```python
from build123d import *

# Parameters (mm, degrees)
SKETCH1_R           = 7.5
BOSS_EXTRUDE1_DEPTH = 300
CUT_EXTRUDE1_DEPTH  = 5


with BuildPart() as part:
    # Sketch1 → Boss-Extrude1 (new body)
    with BuildSketch(Plane.XY):
        with Locations((-21.928145629, 1.412024527)):
            Circle(SKETCH1_R)
    extrude(amount=BOSS_EXTRUDE1_DEPTH)

    # Sketch2 → Cut-Extrude1 (cut)
    with BuildSketch(Plane.XY.offset(300)):
        with BuildLine():
            Line((-23.928145629, 3.412024527), (-23.928145629, -0.587975473))
            ThreePointArc((-23.928145629, -0.587975473), (-21.928145629, -1.587975473), (-19.928145629, -0.587975473))
            Line((-19.928145629, -0.587975473), (-19.928145629, 3.412024527))
            ThreePointArc((-19.928145629, 3.412024527), (-21.928145629, 4.412024527), (-23.928145629, 3.412024527))
        make_face()
    extrude(amount=-CUT_EXTRUDE1_DEPTH, mode=Mode.SUBTRACT)


solid = part.part
```
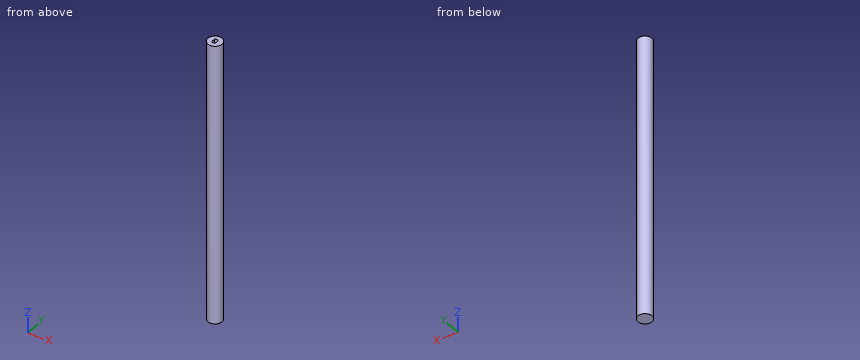
The model under review builds one solid part; all positions refer to its coordinate system, in mm. Round coordinates to 2 decimals unless told otherwise and drop trailing zeros. Write each loop counter-clockwise with the first axis right and the second up, starting at its lowest first coordinate (ties: lowest second). Pieces come first, ordered by that corner, then holes. Notation, with made-up numbers: (23, 65.5) -> (68, 65.5) arc R32 cw to (68, 102.5) -> close; hole circle Ø3 at (-21, -14). An arc over 180 degrees is marked (long way). Use CSV: the item, a comma, the result in double quotes.
Q1. Consider section B-B (z = 158). Give the boundary of the cut face in (x, y).
Checks:
outline,"circle Ø15 at (-21.93, 1.41)"
Q2. For pin 1 Ø4 at (y, z) = (6.5, 49) entering from -X; pin 2 Ø5 at (y, z) = (5.5, 235.5) entering from -X; pin 3 Ø2 at (x, y) = (-22.5, 2.5) entering from +Z, all flat-tipped, find the tip position at first contact; note any pin that passes through.
Checks:
pin 1,"x = -28.76"
pin 2,"x = -29.26"
pin 3,"z = 295"
Q3. To check wall thickness, follow probe 1 along Z at (x, y) = (-21.75, 4); probe 2 along X at (y, z) = (-3.25, 277); probe 3 along Y at (x, z) = (-17, 19). State the ranges of each line that lie inside material, in increasing order. Write a range as [from, to].
Checks:
probe 1,"[0, 295]"
probe 2,"[-27.8, -16.05]"
probe 3,"[-4.24, 7.07]"
Q4. Consider section A-A (x = -17.5). Give the boundary of the cut face in (y, z).
Checks:
outline,"(-4.64, 0) -> (7.47, 0) -> (7.47, 300) -> (-4.64, 300) -> close"
